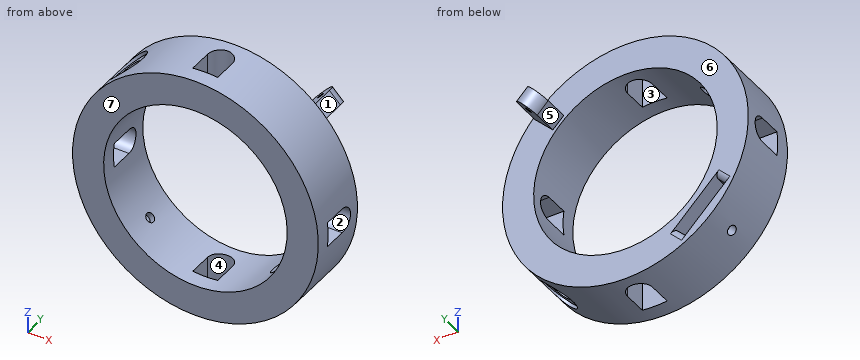
from build123d import *

# Parameters (mm, degrees)
SKETCH1_R               = 39.5
SKETCH1_R_2             = 29.5
BOSS_EXTRUDE1_DEPTH     = 20
CUT_EXTRUDE1_DEPTH      = 60.333801496
CUT_EXTRUDE2_DEPTH      = 60.333801663
CUT_EXTRUDE3_REACH      = 61.334
CUT_EXTRUDE3_END_RADIUS = 39.5
SKETCH4_R               = 3.175
CUT_EXTRUDE4_REACH      = 61.334
CUT_EXTRUDE4_END_RADIUS = 39.5
SKETCH4_2_R             = 3.175
BOSS_EXTRUDE2_DEPTH     = 13
CUT_EXTRUDE7_REACH      = 69.045
CUT_EXTRUDE8_REACH      = 68.559
SKETCH7_R               = 1
SKETCH8_R               = 6.35
CUT_EXTRUDE9_DEPTH      = 1
CUT_EXTRUDE11_DEPTH     = 15
SKETCH10_R              = 1.5
CUT_EXTRUDE12_DEPTH     = 40
FILLET1_R               = 2
FILLET2_R               = 2


with BuildPart() as part:
    # Sketch1 → Boss-Extrude1 (new body)
    with BuildSketch(Plane(origin=(0, 0, 0), x_dir=(1, 0, 0), z_dir=(0, 1, 0))):
        with Locations(Location((0, 0, 0), (0, 0, 270))):
            Circle(SKETCH1_R)
        with Locations(Location((0, 0, 0), (0, 0, 270))):
            Circle(SKETCH1_R_2, mode=Mode.SUBTRACT)
    extrude(amount=BOSS_EXTRUDE1_DEPTH)

    # Sketch2 → Cut-Extrude1 (cut, through all)
    with BuildSketch(Plane(origin=(0, 0, 0), x_dir=(0, 0, -1), z_dir=(1, 0, 0))):
        with BuildLine():
            Line((4, 5), (-4, 5))
            Line((-4, 5), (-4, 12.5))
            ThreePointArc((-4, 12.5), (0, 16.5), (4, 12.5))
            Line((4, 12.5), (4, 5))
        make_face()
    cut_extrude1 = extrude(amount=-CUT_EXTRUDE1_DEPTH, mode=Mode.SUBTRACT)

    # Sketch2<2> → Cut-Extrude2 (cut, through all)
    with BuildSketch(Plane(origin=(0, 0, 0), x_dir=(0, 0, -1), z_dir=(1, 0, 0))):
        with BuildLine():
            Line((4, 5), (-4, 5))
            Line((-4, 5), (-4, 12.5))
            ThreePointArc((-4, 12.5), (0, 16.5), (4, 12.5))
            Line((4, 12.5), (4, 5))
        make_face()
    cut_extrude2 = extrude(amount=CUT_EXTRUDE2_DEPTH, mode=Mode.SUBTRACT)

    # Mirror1: Cut-Extrude1, Cut-Extrude2 across plane
    add(cut_extrude1.mirror(Plane(origin=(0, 0, 0), x_dir=(0.7071067811865478, 0, 0.7071067811865472), z_dir=(0.7071067811865475, 0, -0.7071067811865477))), mode=Mode.SUBTRACT)
    add(cut_extrude2.mirror(Plane(origin=(0, 0, 0), x_dir=(0.7071067811865478, 0, 0.7071067811865472), z_dir=(0.7071067811865475, 0, -0.7071067811865477))), mode=Mode.SUBTRACT)

    # Cut-Extrude3: up to this cylinder (the profile starts inside it)
    cut_extrude3_end = Plane(origin=(0, 10, 0), z_dir=(0, -1, 0)) * Cylinder(CUT_EXTRUDE3_END_RADIUS, 202.668, mode=Mode.PRIVATE)
    # Sketch4 → Cut-Extrude3 (cut, up to the surface)
    with BuildSketch(Plane(origin=(0, 0, 0), x_dir=(-0.7071067811865477, 0, -0.7071067811865475), z_dir=(0.7071067811865475, 0, -0.7071067811865477)), mode=Mode.PRIVATE) as cut_extrude3_sk1:
        with Locations((0, 10)):
            Circle(SKETCH4_R)
    cut_extrude3_tool1 = extrude(cut_extrude3_sk1.sketch, amount=-CUT_EXTRUDE3_REACH, mode=Mode.PRIVATE) & cut_extrude3_end
    add(cut_extrude3_tool1.solids().sort_by_distance((0, 10, 0))[0], mode=Mode.SUBTRACT)

    # Cut-Extrude4: up to this cylinder (the profile starts inside it)
    cut_extrude4_end = Plane(origin=(0, 10, 0), z_dir=(0, -1, 0)) * Cylinder(CUT_EXTRUDE4_END_RADIUS, 202.668, mode=Mode.PRIVATE)
    # Sketch4<2> → Cut-Extrude4 (cut, up to the surface)
    with BuildSketch(Plane(origin=(0, 0, 0), x_dir=(-0.7071067811865477, 0, -0.7071067811865475), z_dir=(0.7071067811865475, 0, -0.7071067811865477)), mode=Mode.PRIVATE) as cut_extrude4_sk1:
        with Locations((0, 10)):
            Circle(SKETCH4_2_R)
    cut_extrude4_tool1 = extrude(cut_extrude4_sk1.sketch, amount=CUT_EXTRUDE4_REACH, mode=Mode.PRIVATE) & cut_extrude4_end
    add(cut_extrude4_tool1.solids().sort_by_distance((0, 10, 0))[0], mode=Mode.SUBTRACT)

    # Sketch5 → Boss-Extrude2 (add)
    with BuildSketch(Plane(origin=(0, 20, 0), x_dir=(1, 0, 0), z_dir=(0, 1, 0))):
        Polygon((25.455844123, -28.991378029), (28.991378029, -25.455844123), (23.334523779, -19.798989873), (19.798989873, -23.334523779), align=None)
    extrude(amount=BOSS_EXTRUDE2_DEPTH)

    # Sketch6 → Cut-Extrude7 (cut, up to next)
    with BuildSketch(Plane(origin=(1.767766953, 0, -1.767766953), x_dir=(-0.7071067811865475, 0, -0.7071067811865477), z_dir=(0.7071067811865477, 0, -0.7071067811865475)), mode=Mode.PRIVATE) as cut_extrude7_sk1:
        with BuildLine():
            Line((-38.5, 28), (-38.5, 33))
            Line((-38.5, 33), (-30.5, 33))
            Line((-30.5, 33), (-30.5, 28))
            ThreePointArc((-30.5, 28), (-34.5, 32), (-38.5, 28))
        make_face()
    cut_extrude7_tool1 = extrude(cut_extrude7_sk1.sketch, amount=-CUT_EXTRUDE7_REACH, mode=Mode.PRIVATE) & part.part
    add(cut_extrude7_tool1.solids().sort_by_distance((26.162951, 32.09434, 22.627417))[0], mode=Mode.SUBTRACT)

    # Sketch7 → Cut-Extrude8 (cut, up to next)
    with BuildSketch(Plane(origin=(1.767766953, 0, -1.767766953), x_dir=(-0.7071067811865475, 0, -0.7071067811865477), z_dir=(0.7071067811865477, 0, -0.7071067811865475)), mode=Mode.PRIVATE) as cut_extrude8_sk1:
        with Locations((-34.5, 28)):
            Circle(SKETCH7_R)
    cut_extrude8_tool1 = extrude(cut_extrude8_sk1.sketch, amount=-CUT_EXTRUDE8_REACH, mode=Mode.PRIVATE) & part.part
    add(cut_extrude8_tool1.solids().sort_by_distance((26.162951, 28, 22.627417))[0], mode=Mode.SUBTRACT)

    # Sketch8 → Cut-Extrude9 (cut)
    with BuildSketch(Plane(origin=(27.930717857, 0, -27.930717857), x_dir=(-0.7071067811865477, 0, -0.7071067811865475), z_dir=(0.7071067811865475, 0, -0.7071067811865477))):
        with Locations((0, 10)):
            Circle(SKETCH8_R)
    cut_extrude9 = extrude(amount=-CUT_EXTRUDE9_DEPTH, mode=Mode.SUBTRACT)

    # Mirror3: Cut-Extrude9 across plane
    add(cut_extrude9.mirror(Plane(origin=(0, 0, 0), x_dir=(0.7071067811865478, 0, 0.7071067811865472), z_dir=(0.7071067811865475, 0, -0.7071067811865477))), mode=Mode.SUBTRACT)

    # Sketch9 → Cut-Extrude11 (cut)
    with BuildSketch(Plane(origin=(0, 20, 0), x_dir=(1, 0, 0), z_dir=(0, 1, 0))):
        Polygon((-19.445436483, 32.173358544), (-32.173358544, 19.445436483), (-28.637824638, 15.909902577), (-15.909902577, 28.637824638), align=None)
    extrude(amount=-CUT_EXTRUDE11_DEPTH, mode=Mode.SUBTRACT)

    # Sketch10 → Cut-Extrude12 (cut)
    with BuildSketch(Plane(origin=(0, 0, 0), x_dir=(0.7071067811865477, 0, -0.7071067811865475), z_dir=(0.7071067811865475, 0, 0.7071067811865477))):
        with Locations((0, 10)):
            Circle(SKETCH10_R)
    extrude(amount=-CUT_EXTRUDE12_DEPTH, mode=Mode.SUBTRACT)

    # Fillet1
    fillet1_edges = [part.edges().sort_by_distance(p)[0] for p in [
        (-17.67766953, 20, -30.405591591),
    ]]
    fillet(fillet1_edges, radius=FILLET1_R)

    # Fillet2
    fillet2_edges = [part.edges().sort_by_distance(p)[0] for p in [
        (-30.405591591, 20, -17.67766953),
    ]]
    fillet(fillet2_edges, radius=FILLET2_R)


solid = part.part
Check sheet for the modelled part. Datum: model origin and axes. Units: mm. Face numbers are marked on the shaded views. A direction names the side the tool comes from. Round coordinates to 2 decimals unless told otherwise and drop trailing zeros. Loops run counter-clockwise (first coordinate to the right, second up) from the corner with the lowest first, then second, coordinate; pieces in that order, holes last. Notation, with made-up numbers: (-21.75, 86) -> (20.25, 86) arc R33 ccw to (20.25, 122) -> close; hole circle Ø2 at (51, -24.75). An arc over 180 degrees is marked (long way). Put each result on its own line as item: value. Start each with the question number.
1. Gauge pin test, flat ends, axial feed: pin 1 (6 mm diameter, centred on y = 7.5, z = -34.5, fed in from -X); pin 2 (4 mm diameter, centred on x = 35, y = 7, fed in from -Z); pin 3 (6 mm diameter, centred on y = 8, z = -33.5, fed in from +X). Record the tip position at first contact, or that the pin passes through.
2. Section check D-D (z = 10.5). Enter the section's corners in (x, y).
3. Section check C-C (z = 0). Enter the section's corners in (x, y).
4. Scan lines: probe 1 along Y at (x, z) = (7.5, 30); probe 2 along X at (y, z) = (10.5, -17); probe 3 along X at (y, z) = (10.5, -31.5). Record each from-to range of solid material in increasing order.
5. Section check A-A (x = 0). Enter the section's corners in (y, z).
6. Access from +Z, -Z, +X, -X, +Y, -Y to the whole of each face (thin tool, end or side, straight path). Record for the marked faces 1, 2 and 3.
7. Draft check along Y on the marked faces 4, 5, 6 and 7. Enter one of: +Y half, -Y half, draft (parallel to the pull), parting line (faces both ways), or undercut.
8. Section check B-B (y = 15). Enter the section's corners in (x, z).
Findings:
1. pin 1: stops at x = -23.83
1. pin 2: stops at z = -21.71
1. pin 3: stops at x = 24.19
2. outline: (-38.08, 0) -> (-27.57, 0) -> (-27.57, 20) -> (-38.08, 20) -> close; (27.57, 0) -> (38.08, 0) -> (38.08, 20) -> (27.57, 20) -> close
3. outline: (-39.5, 0) -> (-29.5, 0) -> (-29.5, 5) -> (-39.5, 5) -> close; (-39.5, 16.5) -> (-29.5, 16.5) -> (-29.5, 20) -> (-39.5, 20) -> close; (29.5, 0) -> (39.5, 0) -> (39.5, 5) -> (29.5, 5) -> close; (29.5, 16.5) -> (39.5, 16.5) -> (39.5, 20) -> (29.5, 20) -> close
4. probe 1: y = 0 to 20
4. probe 2: x = -35.65 to -29.73, -27.55 to -24.11, 24.11 to 35.65
4. probe 3: x = -23.83 to -20.12, -18.77 to -4, 4 to 22.95
5. outline: (0, -39.5) -> (5, -39.5) -> (5, -29.5) -> (0, -29.5) -> close; (0, 29.5) -> (5, 29.5) -> (5, 39.5) -> (0, 39.5) -> close; (16.5, -39.5) -> (20, -39.5) -> (20, -29.5) -> (16.5, -29.5) -> close; (16.5, 29.5) -> (20, 29.5) -> (20, 39.5) -> (16.5, 39.5) -> close
6. face 1: +Z, +X, +Y
6. face 2: +X, -X
6. face 3: +Z, -Z
7. face 4: undercut
7. face 5: draft
7. face 6: +Y half
7. face 7: -Y half
8. outline: (-39.38, -3.12) arc R39.5 ccw to (-3.12, -39.38) -> (-3.12, -29.33) arc R29.5 cw to (-29.33, -3.12) -> close; (-39.38, 3.12) -> (-29.33, 3.12) arc R29.5 cw to (-3.12, 29.33) -> (-3.12, 39.38) arc R39.5 ccw to (-25.03, 30.56) -> (-24.46, 29.99) -> (-29.99, 24.46) -> (-30.56, 25.03) arc R39.5 ccw to start; (3.12, -39.38) arc R39.5 ccw to (25.03, -30.56) -> (24.46, -29.99) -> (29.99, -24.46) -> (30.56, -25.03) arc R39.5 ccw to (39.38, -3.12) -> (29.33, -3.12) arc R29.5 cw to (3.12, -29.33) -> close; (3.12, 29.33) arc R29.5 cw to (29.33, 3.12) -> (39.38, 3.12) arc R39.5 ccw to (3.12, 39.38) -> close; hole (-32.17, -19.45) -> (-19.45, -32.17) -> (-15.91, -28.64) -> (-28.64, -15.91) -> close
